Source: CAD feature listing. Evaluate the final solid. Frame: model axes, mm. Face numbers are marked on the shaded views. A direction names the side the tool comes from. Give positions to 0.01 mm unless a question says otherwise; leave off trailing zeros. Loops run counter-clockwise (first coordinate to the right, second up) from the corner with the lowest first, then second, coordinate; pieces in that order, holes last. Notation, with made-up numbers: (36, 53) -> (84, 53) arc R4 ccw to (84, 60) -> close; hole circle Ø1 at (88.5, 37). An arc over 180 degrees is marked (long way). Put each result on its own line as item: value.
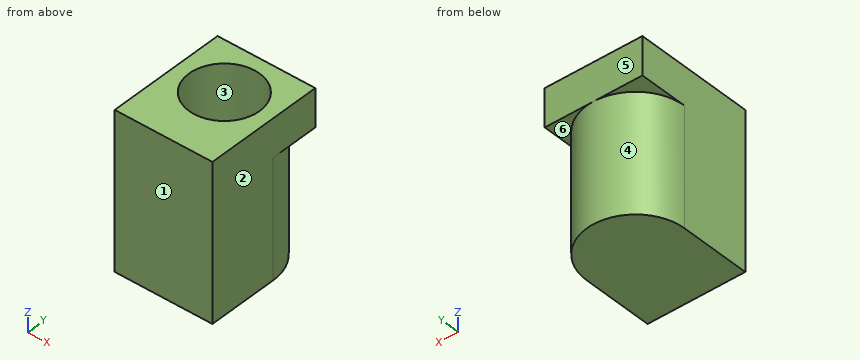
Autodesk Inventor part; units mm, degrees
ref_plane "YZ Plane" through (0, 0, 0) normal (1, 0, 0) x (0, 1, 0)
ref_plane "XZ Plane" through (0, 0, 0) normal (0, 1, 0) x (-1, 0, 0)
ref_plane "XY Plane" through (0, 0, 0) normal (0, 0, 1) x (1, 0, 0)
sketch "Sketch1" plane through (0, 0, 0) normal (0, 0, 1) x (1, 0, 0)
  line L0 (-4.5, 0) -> (4.5, 0)
  line L1 (4.5, 0) -> (4.5, 11)
  line L2 (4.5, 11) -> (-4.5, 11)
  line L3 (-4.5, 11) -> (-4.5, 0)
  line L4 (-4.5, 0) -> (4.5, 11) construction
  line L5 (4.5, 0) -> (-4.5, 11) construction
  point P0 (0, 0)
  point P1 (0, 5.5)
  dimension "d0" = 9
  dimension "d1" = 11
  dimension "d2" = 0
  dimension "d3" = 0
extrude "Extrusion1" add sketch "Sketch1" against normal blind 3.5
sketch "Sketch2" plane through (0, 0, -3.5) normal (0, 0, -1) x (-1, 0, 0)
  line L0 (-4.5, 0) -> (4.5, 0)
  line L1 (4.5, 0) -> (4.5, 11)
  line L2 (4.5, 11) -> (-4.5, 11)
  line L3 (-4.5, 11) -> (-4.5, 0)
  arc A0 (4.5, 6.5) -> (-4.5, 6.5) centre (0, 6.5) ccw
  point P0 (0, 0)
extrude "Extrusion2" add sketch "Sketch2" along normal blind 10.9 contours L3 A0 L1 L0
sketch "Sketch3" plane through (0, 0, 0) normal (0, 0, 1) x (1, 0, 0)
  circle A0 centre (0, 6.5) radius 3.25
  point P0 (0, 0)
  dimension "d8" = 6.5
  dimension "d9" = 6.5
extrude "Extrusion3" cut sketch "Sketch3" against normal blind 10.9
properties part number "pj-002b"
(1) Draft query along Y for the marked faces 1, 2, 3 and 4. Return one class per face: released by +Y, released by -Y, zero draft, split by the parting line, or undercut.
Calculated:
face 1: released by -Y
face 2: zero draft
face 3: undercut
face 4: released by +Y
(2) Section A-A on z = -10.5. Return loops of the section in (x, y).
Calculated:
outline: (-4.5, 0) -> (4.5, 0) -> (4.5, 6.5) arc R4.5 ccw to (-4.5, 6.5) -> close; hole circle Ø6.5 at (0, 6.5)
(3) Line query: probe 1 along Y at (x, z) = (0, -4.75); probe 2 along Z at (x, y) = (-2.75, 6.5); probe 3 along X at (y, z) = (8, -10.25). Output: solid intervals per line, ascending. Write a range as from..to.
Calculated:
probe 1: y = 0..3.25, 9.75..11
probe 2: z = -14.4..-10.9
probe 3: x = -4.24..-2.88, 2.88..4.24
(4) Section B-B on x = 0.75. Return loops of the section in (y, z).
Calculated:
outline: (0, -14.4) -> (10.94, -14.4) -> (10.94, -3.5) -> (11, -3.5) -> (11, 0) -> (9.66, 0) -> (9.66, -10.9) -> (3.34, -10.9) -> (3.34, 0) -> (0, 0) -> close
(5) First-contact query: P1, Ø2, axis at x = 0, y = 7.5, coming from the +Z side; P2, Ø3, axis at x = -2, z = -9.5, coming from the +Y side. Flat tips, straight axial feed; report the tip coordinate or a pass-through.
Calculated:
P1: stops at z = -10.9
P2: stops at y = 10.97
(6) Section D-D on x = 2.25. Return loops of the section in (y, z), then the cut area to 3 significant figures.
Calculated:
outline: (0, -14.4) -> (10.4, -14.4) -> (10.4, -3.5) -> (11, -3.5) -> (11, 0) -> (8.85, 0) -> (8.85, -10.9) -> (4.15, -10.9) -> (4.15, 0) -> (0, 0) -> close
area: 101 mm²
(7) Reachability of the marked faces 5 and 6 from +Z, -Z, +X, -X, +Y, -Y: full face, straight path, thin tool, end or side. Return the list, or none.
Calculated:
face 5: +Z, -Z, +X, -X, +Y
face 6: -Z, +X, +Y
(8) Section C-C on y = 9.25. Return loops of the section in (x, z), then the cut area to 3 significant figures.
Calculated:
outline: (-4.5, -3.5) -> (-3.56, -3.5) -> (-3.56, -14.4) -> (3.56, -14.4) -> (3.56, -3.5) -> (4.5, -3.5) -> (4.5, 0) -> (1.73, 0) -> (1.73, -10.9) -> (-1.73, -10.9) -> (-1.73, 0) -> (-4.5, 0) -> close
area: 71.4 mm²
